Verification items for this drawing (mm, ordinates from the low corner). A direction names the side the tool comes from. Round coordinates to 2 decimals unless told otherwise and drop trailing zeros. Loops run counter-clockwise (first coordinate to the right, second up) from the corner with the lowest first, then second, coordinate; pieces in that order, holes last. Notation, with made-up numbers: (34.25, -20.75) -> (60.25, -20.75) arc R22 ccw to (60.25, 9.25) -> close; hole circle Ø2 at (-33, 3). An arc over 180 degrees is marked (long way). One line per item, written item: value. Start each with the question number.
1. Cross-section at B-B on z = 69.5. Record the cut outline in (x, y), then the cut area to 3 significant figures.
2. Set-up check for the marked faces 4, 5 and 6: record each of +Z, -Z, +X, -X, +Y, -Y from which the full face is reachable in a straight line by a thin tool's end or side.
3. Material ranges on L1, parallel to X at y = 31, z = 26; L2, parallel to Z at x = 60.5, y = 48; L3, parallel to X at y = 9.5, z = 56.5, recorded low to high.
4. Cross-section at D-D on y = 52.5. Record the cut outline in (x, z).
5. Release check for a two-part mould opening along X. For the marked faces 1, 2 and 3 record: +X half, -X half, draft (parallel to the pull), parting line (faces both ways), or undercut.
6. Cross-section at C-C on z = 6. Record the cut outline in (x, y).
7. Go/stop test with flat-tipped pins: pin 1 (8 mm diameter, centred on x = 68, z = 51.5, fed in from +Y); pin 2 (9 mm diameter, centred on x = 85.5, z = 34, fed in from -Y); pin 3 (6 mm diameter, centred on x = 47, z = 18.5, fed in from -Y). Record where each tip stops, or that it passes through.
8. Cross-section at A-A on y = 27. Record the cut outline in (x, z).
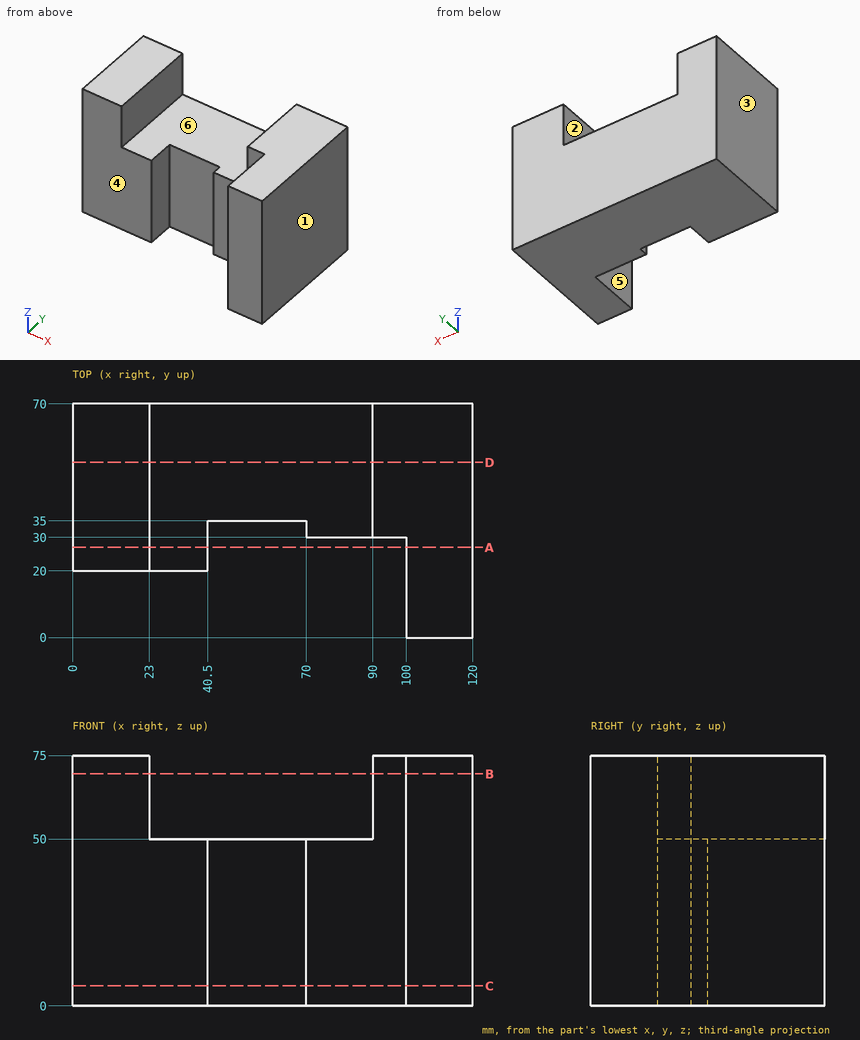
Taken from the geometry:
1. outline: (0, 20) -> (23, 20) -> (23, 70) -> (0, 70) -> close; (90, 30) -> (100, 30) -> (100, 0) -> (120, 0) -> (120, 70) -> (90, 70) -> close
1. area: 2,950 mm2
2. face 4: +Z, -Z, -X, -Y
2. face 5: +Z, -Z, -Y
2. face 6: +Z, +Y, -Y
3. L1: x = 0 to 40.5, 70 to 120
3. L2: z = 0 to 50
3. L3: x = 100 to 120
4. outline: (0, 0) -> (120, 0) -> (120, 75) -> (90, 75) -> (90, 50) -> (23, 50) -> (23, 75) -> (0, 75) -> close
5. face 1: +X half
5. face 2: undercut
5. face 3: -X half
6. outline: (0, 20) -> (40.5, 20) -> (40.5, 35) -> (70, 35) -> (70, 30) -> (100, 30) -> (100, 0) -> (120, 0) -> (120, 70) -> (0, 70) -> close
7. pin 1: stops at y = 70
7. pin 2: stops at y = 30
7. pin 3: stops at y = 35
8. outline: (0, 0) -> (40.5, 0) -> (40.5, 50) -> (23, 50) -> (23, 75) -> (0, 75) -> close; (100, 0) -> (120, 0) -> (120, 75) -> (100, 75) -> close
